Build history of the part. All positions in model axes, mm. Face numbers are marked on the shaded views. A direction names the side the tool comes from. Round coordinates to 2 decimals unless told otherwise and drop trailing zeros. Order: outer loops, then holes, each group sorted by start corner. A loop starts at its lowest first (then second) coordinate and runs counter-clockwise, first axis right, second up. Notation, with made-up numbers: (11.5, 16) -> (67.5, 16) arc R22 ccw to (67.5, 54) -> close; hole circle Ø5 at (50, -7.5). An arc over 180 degrees is marked (long way). Use a Markdown table: item, result. Add a question column.
Item 1: Slice it at D-D, the plane y = -1.6. Give the cut face in (x, z), plus the area to 3 significant figures.
Item 2: Pin check, flat tips, straight feed: pin 1 (1 mm diameter, centred on y = 0, z = -0.5, fed in from -X); pin 2 (3 mm diameter, centred on x = 8, z = -1, fed in from +Y); pin 3 (1 mm diameter, centred on x = 1, z = 2, fed in from +Y). Stop position of each tip, or through.
Item 3: Slice it at B-B, the plane z = 0.25. Give the cut face in (x, y), plus the area to 3 significant figures.
Item 4: Probe L1, parallel to X at y = 0.3, z = -1; L2, parallel to X at y = 0.7, z = 1.7; L3, parallel to Y at x = 0.5, z = -0.1. List the from-to ranges inside material, lowest first.
Item 5: Two-plate mould, pull along Y, no slides. Class the marked faces 3, 4 and 5: released by +Y, released by -Y, zero draft, split by the parting line, or undercut.
Item 6: Slice it at A-A, the plane y = 0. Give the cut face in (x, z).
Item 7: Slice it at C-C, the plane x = 5. Give the cut face in (y, z), plus the area to 3 significant figures.
Item 8: 3-axis set-ups, long thin cutter, end or side, ignore diameter. For the marked faces 1 and 2: which of +Z, -Z, +X, -X, +Y, -Y reach the whole face in a straight line?
from build123d import *

# Parameters (mm, degrees)
SKETCH1_R             = 1.75
THREADED_SCREW_DEPTH  = 10
SKETCH2_R             = 2.75
ROUND_HEAD_DEPTH      = 3
HEX_SOCKET_SIZE_DEPTH = 2


with BuildPart() as part:
    # Sketch1 → Threaded_Screw (new body)
    with BuildSketch(Plane(origin=(0, 0, 0), x_dir=(0, 0, -1), z_dir=(1, 0, 0))):
        Circle(SKETCH1_R)
    extrude(amount=THREADED_SCREW_DEPTH)

    # Sketch2 → Round_Head (add)
    with BuildSketch(Plane.ZY):
        Circle(SKETCH2_R)
    extrude(amount=ROUND_HEAD_DEPTH)

    # Sketch3 → Hex_Socket_Size (cut)
    with BuildSketch(Plane.ZY.offset(3)):
        Polygon((1.25, -0.721687836), (1.25, 0.721687836), (0, 1.443375673), (-1.25, 0.721687836), (-1.25, -0.721687836), (0, -1.443375673), align=None)
    extrude(amount=-HEX_SOCKET_SIZE_DEPTH, mode=Mode.SUBTRACT)


solid = part.part
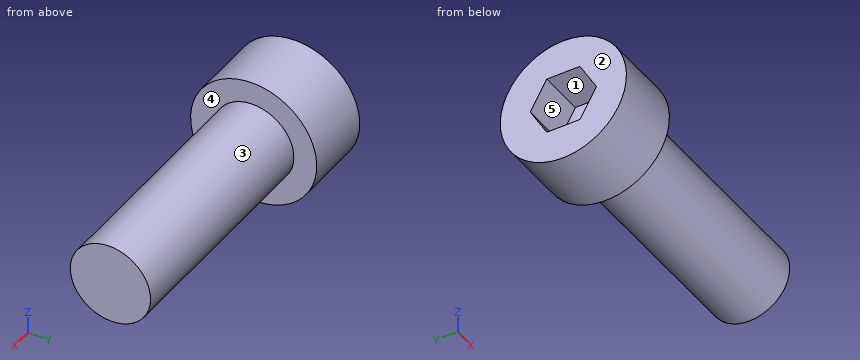
Check sheet entries:
| question | item | result |
|---|---|---|
| 1 | outline | (-3, -2.24) -> (0, -2.24) -> (0, -0.71) -> (10, -0.71) -> (10, 0.71) -> (0, 0.71) -> (0, 2.24) -> (-3, 2.24) -> close |
| 1 | area | 27.6 mm2 |
| 2 | pin 1 | x = -1 |
| 2 | pin 2 | y = 1.75 |
| 2 | pin 3 | y = 0.9 |
| 3 | outline | (-3, -2.74) -> (0, -2.74) -> (0, -1.73) -> (10, -1.73) -> (10, 1.73) -> (0, 1.73) -> (0, 2.74) -> (-3, 2.74) -> (-3, 1.3) -> (-1, 1.3) -> (-1, -1.3) -> (-3, -1.3) -> close |
| 3 | area | 45.9 mm2 |
| 4 | L1 | -1 to 10 |
| 4 | L2 | -3 to 0 |
| 4 | L3 | -1.75 to 1.75 |
| 5 | face 3 | split by the parting line |
| 5 | face 4 | zero draft |
| 5 | face 5 | undercut |
| 6 | outline | (-3, -2.75) -> (0, -2.75) -> (0, -1.75) -> (10, -1.75) -> (10, 1.75) -> (0, 1.75) -> (0, 2.75) -> (-3, 2.75) -> (-3, 1.25) -> (-1, 1.25) -> (-1, -1.25) -> (-3, -1.25) -> close |
| 7 | outline | circle Ø3.5 at (0, 0) |
| 7 | area | 9.62 mm2 |
| 8 | face 1 | -X |
| 8 | face 2 | +Z, -Z, -X, +Y, -Y |
